CAD build for the part. Positions are in the model's coordinates, mm. A direction names the side the tool comes from. Coordinates: 2 decimals unless noted, no trailing zeros. Order: outer loops, then holes, each group sorted by start corner. A loop starts at its lowest first (then second) coordinate and runs counter-clockwise, first axis right, second up. Notation, with made-up numbers: (77, 8) - (127, 8) arc R14 ccw to (127, 21) - close; hole circle Ø6 at (-10.5, -23.5). An arc over 180 degrees is marked (long way). Return JSON: item names as keys, results as strings.
from build123d import *

# Parameters (mm, degrees)
SKETCH_W        = 80
SKETCH_H        = 110
PAD_DEPTH       = 5
SKETCH001_W     = 8
SKETCH001_H     = 3.5
PAD001_DEPTH    = 20
SKETCH002_W     = 59
SKETCH002_H     = 26
PAD002_DEPTH    = 50
SKETCH003_W     = 40.3
SKETCH003_H     = 20.5
POCKET_DEPTH    = 55.001
SKETCH004_W     = 5.2
SKETCH004_H     = 50
POCKET001_DEPTH = 10
SKETCH005_R     = 1
POCKET002_DEPTH = 10
SKETCH006_W     = 17.7
SKETCH006_H     = 10.9
SKETCH006_W_2   = 12.7
SKETCH006_H_2   = 5.9
PAD003_DEPTH    = 12
SKETCH007_W     = 8
SKETCH007_H     = 3.5
POCKET003_DEPTH = 20
POCKET004_DEPTH = 5
POCKET005_DEPTH = 5
POCKET006_DEPTH = 26
POCKET007_DEPTH = 5
FILLET_R        = 5
FILLET001_R     = 5
SKETCH012_R     = 2.25
POCKET008_DEPTH = 5


with BuildPart() as part:
    # Sketch → Pad (new body)
    with BuildSketch(Plane.XY):
        Rectangle(SKETCH_W, SKETCH_H)
    extrude(amount=PAD_DEPTH)

    # Sketch001 (on Face6 of Pad) → Pad001 (join)
    with BuildSketch(Plane.XY.offset(5)):
        with Locations((1, 47.75)):
            Rectangle(SKETCH001_W, SKETCH001_H)
        with Locations((1, -47.75)):
            Rectangle(SKETCH001_W, SKETCH001_H)
    extrude(amount=PAD001_DEPTH)

    # Sketch002 (on Face5 of Pad001) → Pad002 (join)
    with BuildSketch(Plane.XY.offset(5)):
        with Locations((1.5, -4)):
            Rectangle(SKETCH002_W, SKETCH002_H)
    extrude(amount=PAD002_DEPTH)

    # Sketch003 (on Face4 of Pad002) → Pocket (cut, through all)
    with BuildSketch(Plane(origin=(0, 0, 0), x_dir=(1, 0, 0), z_dir=(0, 0, -1))):
        with Locations((1.5, 4)):
            Rectangle(SKETCH003_W, SKETCH003_H)
    extrude(amount=-POCKET_DEPTH, mode=Mode.SUBTRACT)

    # Sketch004 (on Face17 of Pocket) → Pocket001 (cut)
    with BuildSketch(Plane.YZ.offset(31)):
        with Locations((-4, 30)):
            Rectangle(SKETCH004_W, SKETCH004_H)
    extrude(amount=-POCKET001_DEPTH, mode=Mode.SUBTRACT)

    # Sketch005 (on Face25 of Pocket001) → Pocket002 (cut)
    with BuildSketch(Plane.XY.offset(55)):
        with Locations((-23, 0.8)):
            Circle(SKETCH005_R)
        with Locations((-23, -8.8)):
            Circle(SKETCH005_R)
        with Locations((26, -8.8)):
            Circle(SKETCH005_R)
        with Locations((26, 0.8)):
            Circle(SKETCH005_R)
    extrude(amount=-POCKET002_DEPTH, mode=Mode.SUBTRACT)

    # Sketch006 (on Face5 of Pocket002) → Pad003 (join)
    with BuildSketch(Plane.XY.offset(5)):
        with Locations((1, 47.75)):
            Rectangle(SKETCH006_W, SKETCH006_H)
        with Locations((1, 47.75)):
            Rectangle(SKETCH006_W_2, SKETCH006_H_2, mode=Mode.SUBTRACT)
        with Locations((1, -47.75)):
            Rectangle(SKETCH006_W, SKETCH006_H)
        with Locations((1, -47.75)):
            Rectangle(SKETCH006_W_2, SKETCH006_H_2, mode=Mode.SUBTRACT)
    extrude(amount=PAD003_DEPTH)

    # Sketch007 (on Face57 of Pad003) → Pocket003 (cut)
    with BuildSketch(Plane.XY.offset(25)):
        with Locations((1, -47.75)):
            Rectangle(SKETCH007_W, SKETCH007_H)
        with Locations((1, 47.75)):
            Rectangle(SKETCH007_W, SKETCH007_H)
    extrude(amount=-POCKET003_DEPTH, mode=Mode.SUBTRACT)

    # Sketch008 (on Face5 of Pocket003) → Pocket004 (cut)
    with BuildSketch(Plane.XY.offset(5)):
        Polygon((-40, 55), (-10.35, 55), (-40, 10.5), align=None)
        Polygon((-40, -18.5), (-40, -55), (-10.35, -55), align=None)
        Polygon((40, -18.5), (40, -55), (12.35, -55), align=None)
        Polygon((40, 10.5), (40, 55), (12.35, 55), align=None)
    extrude(amount=-POCKET004_DEPTH, mode=Mode.SUBTRACT)

    # Sketch009 (on Face4 of Pocket004) → Pocket005 (cut)
    with BuildSketch(Plane.XY.offset(5)):
        with BuildLine():
            Line((-18.5, 9), (21.5, 9))
            ThreePointArc((21.5, 9), (1.5, 29), (-18.5, 9))
        make_face()
        with BuildLine():
            Line((-18.5, -17), (21.5, -17))
            ThreePointArc((-18.5, -17), (1.5, -37.000028), (21.5, -17))
        make_face()
    extrude(amount=-POCKET005_DEPTH, mode=Mode.SUBTRACT)

    # Sketch010 (on Face27 of Pocket005) → Pocket006 (cut)
    with BuildSketch(Plane(origin=(0, 9, 0), x_dir=(-1, 0, 0), z_dir=(0, 1, 0))):
        with BuildLine():
            Line((-21.5, 5), (-21.5, 25))
            ThreePointArc((18.5, 25), (-1.5, 45), (-21.5, 25))
            Line((18.5, 5), (18.5, 25))
            Line((-21.5, 5), (18.5, 5))
        make_face()
    extrude(amount=-POCKET006_DEPTH, mode=Mode.SUBTRACT)

    # Sketch011 (on Face2 of Pocket006) → Pocket007 (cut)
    with BuildSketch(Plane(origin=(0, 0, 0), x_dir=(1, 0, 0), z_dir=(0, 0, -1))):
        Polygon((-18.5, 17), (-18.65, 14.25), (-18.65, -6.25), (-18.5, -9), (21.5, -9), (21.65, -6.25), (21.65, 14.25), (21.5, 17), align=None)
    extrude(amount=-POCKET007_DEPTH, mode=Mode.SUBTRACT)

    # Fillet
    fillet_edges = [part.edges().sort_by_distance(p)[0] for p in [
        (40, -18.5, 2.5),
        (40, 10.5, 2.5),
        (12.35, -55, 2.5),
        (-10.35, -55, 2.5),
        (-10.35, 55, 2.5),
        (12.35, 55, 2.5),
        (-40, -18.5, 2.5),
        (-40, 10.5, 2.5),
    ]]
    fillet(fillet_edges, radius=FILLET_R)

    # Fillet001
    fillet001_edges = [part.edges().sort_by_distance(p)[0] for p in [
        (-28, -17, 30),
        (-28, 9, 30),
        (31, -17, 30),
        (31, 9, 30),
    ]]
    fillet(fillet001_edges, radius=FILLET001_R)

    # Sketch012 (on Face81 of Fillet001) → Pocket008 (cut)
    with BuildSketch(Plane.XY.offset(5)):
        with Locations((1, 47.75)):
            Circle(SKETCH012_R)
        with Locations((1, -47.75)):
            Circle(SKETCH012_R)
    extrude(amount=-POCKET008_DEPTH, mode=Mode.SUBTRACT)


solid = part.part
Item 1: Drop flat-ended pins along their axis: P1, Ø12, axis at y = -46, z = 12.5, coming from the -X side; P2, Ø6.5, axis at x = 0.5, y = 49, coming from the +Z side; P3, Ø2.5, axis at y = -8.5, z = 18.5, coming from the +X side; P4, Ø1.6, axis at x = 26.5, y = 1, coming from the +Z side. Give the stop position or say it passes through.
Findings below:
{"P1": "stops at x = -7.85", "P2": "stops at z = 17", "P3": "stops at x = 31", "P4": "stops at z = 55"}
Item 2: Band-saw the part on C-C, the plane x = 20. List the corners of the cut face in (y, z), then the cut area to 3 significant figures.
Findings below:
{"outline": "(-44.9, 0) - (-24.6, 0) - (-24.6, 5) - (-44.9, 5) - close; (-17, 32.6) - (-14.25, 32.6) - (-14.25, 55) - (-17, 55) - close; (6.25, 32.6) - (9, 32.6) - (9, 55) - (6.25, 55) - close; (16.6, 0) - (42.69, 0) - (42.69, 5) - (16.6, 5) - close", "area": "355 mm²"}
Item 3: Wall check: L1, parallel to Y at x = 1, z = 2; L2, parallel to Y at x = -23, z = 51; L3, parallel to X at y = -8, z = 39. Give the ranges that are in metal, low to high. Write a range as [from, to].
Findings below:
{"L1": "y = [-55, -50], [-45.5, -36.99], [28.99, 45.5], [50, 55]", "L2": "y = [-17, -9.8], [-7.8, -0.2], [1.8, 9]", "L3": "x = [-28, -18.65], [21.65, 31]"}
Item 4: Mould opens along X. For faces 6 (the cylindrical face through (11.969, 54.387, 2.465)), 7 (the cylindrical face through (-39.72, -18.38, 2.46)), 8 (the flat face through (-18.574, -15.644, 2.465)), 9 (the flat face through (1, -17, 47)) say: released by +X, released by -X, zero draft, split by the parting line, or undercut.
Findings below:
{"face 6": "released by +X", "face 7": "released by -X", "face 8": "undercut", "face 9": "zero draft"}
Item 5: Band-saw the part on D-D, the plane z = 52. List the corners of the cut face in (x, y), then the cut area to 3 significant figures.
Findings below:
{"outline": "(-28, -12) arc R5 ccw to (-23, -17) - (26, -17) arc R5 ccw to (31, -12) - (31, -6.6) - (21.65, -6.6) - (21.65, -14.25) - (-18.65, -14.25) - (-18.65, 6.25) - (21.65, 6.25) - (21.65, -1.4) - (31, -1.4) - (31, 4) arc R5 ccw to (26, 9) - (-23, 9) arc R5 ccw to (-28, 4) - close; hole circle Ø2 at (-23, -8.8); hole circle Ø2 at (-23, 0.8); hole circle Ø2 at (26, -8.8); hole circle Ø2 at (26, 0.8)", "area": "625 mm²"}
Item 6: Band-saw the part on A-A, the plane y = -47.75. List the corners of the cut face in (x, z), then the cut area to 3 significant figures.
Findings below:
{"outline": "(-16.24, 0) - (-1.25, 0) - (-1.25, 5) - (-5.35, 5) - (-5.35, 17) - (-7.85, 17) - (-7.85, 5) - (-16.24, 5) - close; (3.25, 0) - (17.84, 0) - (17.84, 5) - (9.85, 5) - (9.85, 17) - (7.35, 17) - (7.35, 5) - (3.25, 5) - close", "area": "208 mm²"}
Item 7: Which spindle directions (+Z, -Z, +X, -X, +Y, -Y) get a long thin tool onto all of the face, cutting with end or side? Do faces 1 (the flat face through (21.574, 7.644, 2.465)), 2 (the cylindrical face through (1.06, -36.995, 2.535)), 3 (the flat face through (-7.85, -48, 11)), 4 (the flat face through (9.85, 48, 11)), 5 (the flat face through (1, -42.3, 11)). Say none if no direction does.
Findings below:
{"face 1": "-Z", "face 2": "+Z, -Z", "face 3": "+Z, -X, +Y, -Y", "face 4": "+Z, +X, +Y, -Y", "face 5": "+Z, +X, -X"}
Item 8: Band-saw the part on B-B, the plane z = 34. List the corners of the cut face in (x, y), then the cut area to 3 significant figures.
Findings below:
{"outline": "(-28, -12) arc R5 ccw to (-23, -17) - (-16.36, -17) - (-16.36, -14.25) - (-18.65, -14.25) - (-18.65, 6.25) - (-16.36, 6.25) - (-16.36, 9) - (-23, 9) arc R5 ccw to (-28, 4) - close; (19.36, -17) - (26, -17) arc R5 ccw to (31, -12) - (31, -6.6) - (21.65, -6.6) - (21.65, -14.25) - (19.36, -14.25) - close; (19.36, 6.25) - (21.65, 6.25) - (21.65, -1.4) - (31, -1.4) - (31, 4) arc R5 ccw to (26, 9) - (19.36, 9) - close", "area": "441 mm²"}
